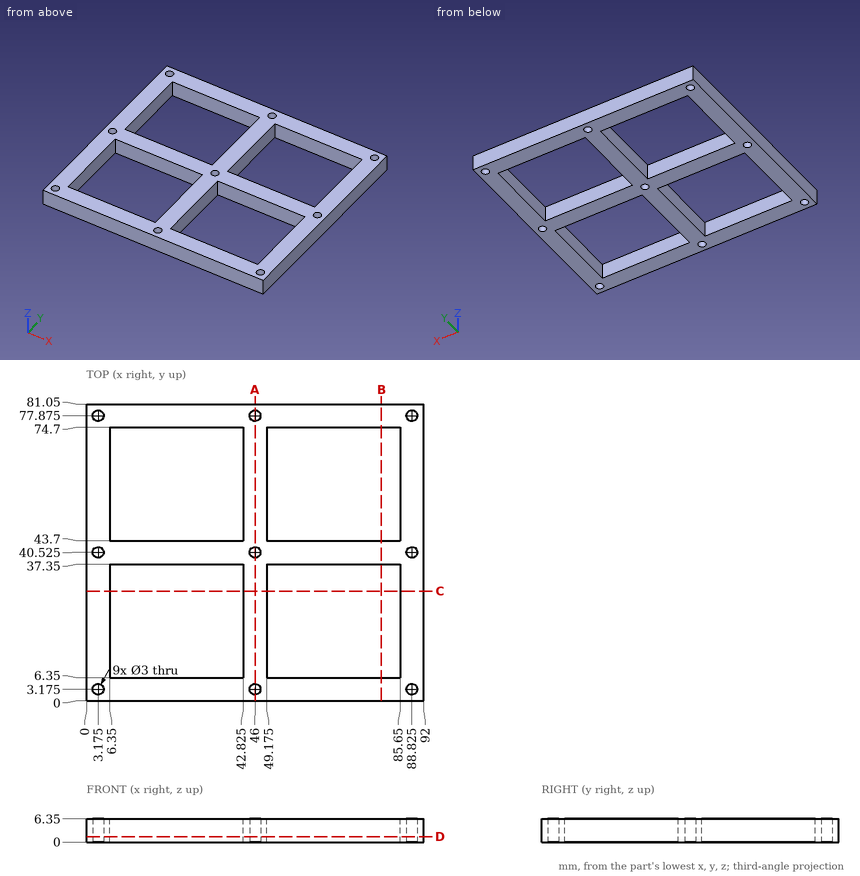
Design review of the part shown in the three views and the two pictorial views. Dimensions are in mm from the part's minimum x, y and z. Round coordinates to 2 decimals unless told otherwise and drop trailing zeros. Write each loop counter-clockwise with the first axis right and the second up, starting at its lowest first coordinate (ties: lowest second). Pieces come first, ordered by that corner, then holes.
Item 1: Wall thickness on L1, parallel to Y at x = 61, z = 5.25; L2, parallel to X at y = 26, z = 4.5 (3 decimals); L3, parallel to X at y = 40, z = 4.5: over which ranges is each line inside the solid? List them lowest first.
Item 2: Consider section D-D on z = 1.5. Count the separate pieces of the cut face and the enclosed holes in it, and give its area (3 significant figures).
Item 3: For pin 1 Ø2.5 at (x, y) = (3.175, 77.875) entering from +Z, flat-tipped, find the tip position at first contact; note if it passes through.
Item 4: Consider section A-A on x = 46. Give the boundary of the cut face in (y, z) (3 decimals), and give its area (3 significant figures).
Item 5: Consider section B-B on x = 80.5. Give the boundary of the cut face in (y, z), and give its area (3 significant figures).
Item 6: Consider section C-C on y = 30. Give the boundary of the cut face in (x, z) (3 decimals).
Check values:
1. L1: y = 0 to 6.35, 37.35 to 43.7, 74.7 to 81.05
1. L2: x = 0 to 6.35, 42.825 to 49.175, 85.65 to 92
1. L3: x = 0 to 1.77, 4.58 to 44.59, 47.41 to 87.42, 90.23 to 92
2. separate pieces: 1
2. enclosed holes: 13
2. area: 2,870 mm2
3. pin 1: passes through
4. outline: (0, 0) - (1.675, 0) - (1.675, 6.35) - (0, 6.35) - close; (4.675, 0) - (39.025, 0) - (39.025, 6.35) - (4.675, 6.35) - close; (42.025, 0) - (76.375, 0) - (76.375, 6.35) - (42.025, 6.35) - close; (79.375, 0) - (81.05, 0) - (81.05, 6.35) - (79.375, 6.35) - close
4. area: 458 mm2
5. outline: (0, 0) - (6.35, 0) - (6.35, 6.35) - (0, 6.35) - close; (37.35, 0) - (43.7, 0) - (43.7, 6.35) - (37.35, 6.35) - close; (74.7, 0) - (81.05, 0) - (81.05, 6.35) - (74.7, 6.35) - close
5. area: 121 mm2
6. outline: (0, 0) - (6.35, 0) - (6.35, 6.35) - (0, 6.35) - close; (42.825, 0) - (49.175, 0) - (49.175, 6.35) - (42.825, 6.35) - close; (85.65, 0) - (92, 0) - (92, 6.35) - (85.65, 6.35) - close
